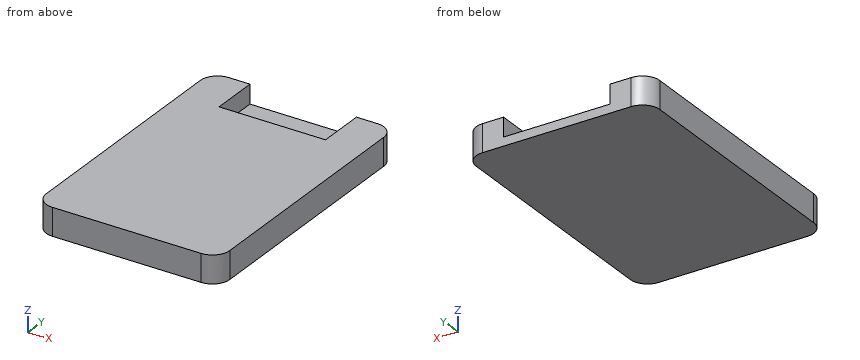
from build123d import *

# Parameters (mm, degrees)
F0_W     = 12.3
F0_H     = 9.7
F1_DEPTH = 3.2
F2_R     = 2
F3_DEPTH = 2.5
F0_H_2   = 5.5
F4_DEPTH = 1


with BuildPart() as f1:
    # F0 (on Top) → F1 (new body)
    with BuildSketch(Plane.XY):
        Polygon((-44.4362910628, 49.737931484), (-48.8862910628, 49.737931484), (-48.8862910628, 18.337931484), (-27.6862910628, 18.337931484), (-27.6862910628, 49.737931484), (-32.1362910628, 49.737931484), (-32.1362910628, 44.237931484), (-32.1362910628, 34.537931484), (-44.4362910628, 34.537931484), (-44.4362910628, 44.237931484), align=None)
        with Locations((-38.2862910628, 39.387931484)):
            Rectangle(F0_W, F0_H)
    extrude(amount=F1_DEPTH)

    # F2
    f2_edges = [f1.edges().sort_by_distance(p)[0] for p in [
        (-27.686291, 18.337931, 1.6),
        (-27.686291, 49.737931, 1.6),
        (-48.886291, 18.337931, 1.6),
        (-48.886291, 49.737931, 1.6),
    ]]
    fillet(f2_edges, radius=F2_R)

    # F0 (on Top) → F3 (cut)
    with BuildSketch(Plane.XY):
        with Locations((-38.2862910628, 39.387931484)):
            Rectangle(F0_W, F0_H)
    extrude(amount=F3_DEPTH, mode=Mode.SUBTRACT)

    # F0 (on Top) → F4 (join)
    with BuildSketch(Plane.XY):
        with Locations((-38.2862910628, 39.387931484)):
            Rectangle(F0_W, F0_H)
        with Locations((-38.2862910628, 46.987931484)):
            Rectangle(F0_W, F0_H_2)
    extrude(amount=F4_DEPTH)


solid = f1.part
The listing builds one solid part. Answer for the finished solid, in the listing's coordinates (mm). Round coordinates to 2 decimals unless told otherwise and drop trailing zeros. Order: outer loops, then holes, each group sorted by start corner. A loop starts at its lowest first (then second) coordinate and runs counter-clockwise, first axis right, second up. Notation, with made-up numbers: (-17.75, -18.5) -> (-6.75, -18.5) arc R26 ccw to (-6.75, 15.5) -> close; hole circle Ø5 at (79.5, 11). An arc over 180 degrees is marked (long way). Put each result on its own line as item: value.
Q1. Section C-C, the plane x = -38 is taken. Write down the section's boundary in (y, z).
Results list:
outline: (18.34, 0) -> (49.74, 0) -> (49.74, 1) -> (34.54, 1) -> (34.54, 2.5) -> (44.24, 2.5) -> (44.24, 3.2) -> (18.34, 3.2) -> close
Q2. This flat-tipped pin is pushed along its axis until it touches: P1, Ø12, axis at x = -40.5, y = 45, coming from the -Z side. Where does it stop, or does it pass through?
Results list:
P1: z = 0
Q3. Section A-A, the plane z = 1.8 is taken. Write down the section's boundary in (x, y).
Results list:
outline: (-48.89, 20.34) arc R2 ccw to (-46.89, 18.34) -> (-29.69, 18.34) arc R2 ccw to (-27.69, 20.34) -> (-27.69, 47.74) arc R2 ccw to (-29.69, 49.74) -> (-32.14, 49.74) -> (-32.14, 34.54) -> (-44.44, 34.54) -> (-44.44, 49.74) -> (-46.89, 49.74) arc R2 ccw to (-48.89, 47.74) -> close
Q4. Section D-D, the plane y = 46 is taken. Write down the section's boundary in (x, z), and give its area (3 significant figures).
Results list:
outline: (-48.89, 0) -> (-27.69, 0) -> (-27.69, 3.2) -> (-32.14, 3.2) -> (-32.14, 1) -> (-44.44, 1) -> (-44.44, 3.2) -> (-48.89, 3.2) -> close
area: 40.8 mm^2
Q5. Consider line 1 along Z through (x, y) = (-37.5, 35); line 2 along X through (y, z) = (43, 1.8); line 3 along Z through (x, y) = (-37, 44.5). Determine where each line is inside the solid, lowest interval first.
Results list:
line 1: 0 to 1, 2.5 to 3.2
line 2: -48.89 to -44.44, -32.14 to -27.69
line 3: 0 to 1
Q6. Section B-B, the plane y = 37.5 is taken. Write down the section's boundary in (x, z).
Results list:
outline: (-48.89, 0) -> (-27.69, 0) -> (-27.69, 3.2) -> (-48.89, 3.2) -> close; hole (-44.44, 1) -> (-32.14, 1) -> (-32.14, 2.5) -> (-44.44, 2.5) -> close
